from build123d import *

# Parameters (mm, degrees)
F0_R     = 7
F0_R_2   = 4.5
F1_DEPTH = 30
F2_DEPTH = 23
F3_R     = 1


with BuildPart() as f1:
    # F0 (on Front) → F1 (new body)
    with BuildSketch(Plane.XZ):
        Circle(F0_R)
        Circle(F0_R_2, mode=Mode.SUBTRACT)
        Circle(F0_R_2)
    extrude(amount=-F1_DEPTH)

    # F0 (on Front) → F2 (join)
    with BuildSketch(Plane.XZ):
        Circle(F0_R_2)
    extrude(amount=F2_DEPTH)

    # F3
    f3_edges = [f1.edges().sort_by_distance(p)[0] for p in [
        (-4.5, -23, 0),
        (-7, 0, 0),
    ]]
    fillet(f3_edges, radius=F3_R)


solid = f1.part
Verification items for the finished model (mm, model axes). A direction names the side the tool comes from. Coordinates: 2 decimals unless noted, no trailing zeros. Order: outer loops, then holes, each group sorted by start corner. A loop starts at its lowest first (then second) coordinate and runs counter-clockwise, first axis right, second up. Notation, with made-up numbers: M 50.5,18 L 87.5,18 A26 cw 87.5,49 Z; hole C 3,-20 d6. An arc over 180 degrees is marked long. One line per item, written item: value. Start each with the question number.
Item 1: Sectioned sample at A-A on x = 0. Record the cut outline in (y, z).
Item 2: Depth check by flat-ended pin: P1, Ø2, axis at x = 4.5, y = -9.5, coming from the -Z side; P2, Ø2, axis at x = -2, y = -7.5, coming from the -Z side; P3, Ø1.5, axis at x = -1, y = -15, coming from the -Z side. Enter the tip coordinate at first touch or a pass-through.
Item 3: Sectioned sample at D-D on y = -1.5. Record the cut outline in (x, z), then the cut area to 3 significant figures.
Item 4: Sectioned sample at B-B on z = 0. Record the cut outline in (x, y).
Item 5: Thickness scan on probe 1 along Y at (x, z) = (4.75, -1); probe 2 along X at (y, z) = (-10, 0.25); probe 3 along X at (y, z) = (9, -4.5). Record the ranges inside material, lowest first.
Item 6: Access from +Z, -Z, +X, -X, +Y, -Y to the whole of each face (thin tool, end or side, straight path). Record for faces 1 (the flat face through (0, -23, 0)), 2 (the cylindrical face through (-0.59, -10.85, 4.46)).
Item 7: Sectioned sample at C-C on y = 19. Record the cut outline in (x, z).
Item 8: Mould release check, pull along Z, two halves, no side actions. Record for faces 3 (the flat face through (-1.4, 0, 4.5)), 4 (the cylindrical face through (6.466, 15.297, -2.681)): pulls with the +Z half, pulls with the -Z half, needs draft (parallel to the pull), parting line crosses it, or undercut.
Calculated:
1. outline: M -23,-3.5 A1 ccw -22,-4.5 L 0,-4.5 L 0,-6 A1 ccw 1,-7 L 30,-7 L 30,7 L 1,7 A1 ccw 0,6 L 0,4.5 L -22,4.5 A1 ccw -23,3.5 Z
2. P1: z = -2.83
2. P2: z = -4.39
2. P3: z = -4.49
3. outline: C 0,0 d9
3. area: 63.6 mm^2
4. outline: M -7,1 A1 ccw -6,0 L -4.5,0 L -4.5,-22 A1 ccw -3.5,-23 L 3.5,-23 A1 ccw 4.5,-22 L 4.5,0 L 6,0 A1 ccw 7,1 L 7,30 L -7,30 Z
5. probe 1: 0 to 30
5. probe 2: -4.49 to 4.49
5. probe 3: -5.36 to 5.36
6. face 1: +Z, -Z, +X, -X, -Y
6. face 2: -Y
7. outline: C 0,0 d14
8. face 3: needs draft
8. face 4: parting line crosses it
